from build123d import *

# Parameters (mm, degrees)
F0_W     = 108.1513464451
F0_H     = 106.336735189
F1_DEPTH = 25.4
F2_R     = 30.7442953742
F3_DEPTH = 25.401
F4_R     = 45.0892018552
F4_R_2   = 30.7442953742
F5_DEPTH = 25.4


with BuildPart() as f1:
    # F0 (on Front) → F1 (new body)
    with BuildSketch(Plane.XZ):
        Rectangle(F0_W, F0_H)
    extrude(amount=F1_DEPTH)

    # F2 (on face) → F3 (cut, through all)
    with BuildSketch(Plane.XZ.offset(25.4)):
        Circle(F2_R)
    extrude(amount=-F3_DEPTH, mode=Mode.SUBTRACT)

    # F4 (on face) → F5 (join)
    with BuildSketch(Plane.XZ.offset(25.4)):
        Circle(F4_R)
        Circle(F4_R_2, mode=Mode.SUBTRACT)
    extrude(amount=F5_DEPTH)


solid = f1.part
Part model, mm, in its own coordinate system. A direction names the side the tool comes from. Round coordinates to 2 decimals unless told otherwise and drop trailing zeros. Write each loop counter-clockwise with the first axis right and the second up, starting at its lowest first coordinate (ties: lowest second). Pieces come first, ordered by that corner, then holes. Notation, with made-up numbers: M 14,13 L 26,13 A26 cw 26,41 Z; hole C 63,64.25 d7. An arc over 180 degrees is marked long. Return JSON: item names as keys, results as strings. Group by question number.
(1) Drill centre lines: probe 1 along Z at (x, y) = (0, -40.25); probe 2 along X at (y, z) = (-37, 1); probe 3 along Z at (x, y) = (0, -11). Where is each one in solid material? Low to high.
(2) Which spindle directions (+Z, -Z, +X, -X, +Y, -Y) get a long thin tool onto all of the face, cutting with end or side? Do faces 1 (the face through (-1, -25.4, -47)), 2 (the face through (54.076, -13, -1)). Say none if no direction does.
(3) Saw through at B-B on z = 0. Write the cut outline in (x, y).
(4) Saw through at C-C on y = -16. Write the cut outline in (x, z), then the cut area to 3 significant figures.
(5) Pin check, flat tips, straight feed: pin 1 Ø8 at (y, z) = (-41.5, -11) entering from +X; pin 2 Ø1.5 at (x, y) = (14, -40.5) entering from -Z; pin 3 Ø2 at (y, z) = (-41, 27.5) entering from -X. Stop position of each tip, or through.
(6) Saw through at D-D on z = 39. Write the cut outline in (x, y).
(7) Saw through at A-A on x = 0. Write the cut outline in (y, z).
Returned:
{
 "1": {"probe 1": "-45.09 to -30.74, 30.74 to 45.09", "probe 2": "-45.08 to -30.73, 30.73 to 45.08", "probe 3": "-53.17 to -30.74, 30.74 to 53.17"},
 "2": {"face 1": "-Y", "face 2": "+Z, -Z, +X, +Y, -Y"},
 "3": {"outline": "M -54.08,-25.4 L -45.09,-25.4 L -45.09,-50.8 L -30.74,-50.8 L -30.74,0 L -54.08,0 Z; M 30.74,-50.8 L 45.09,-50.8 L 45.09,-25.4 L 54.08,-25.4 L 54.08,0 L 30.74,0 Z"},
 "4": {"outline": "M -54.08,-53.17 L 54.08,-53.17 L 54.08,53.17 L -54.08,53.17 Z; hole C 0,0 d61.49", "area": "8,530 mm²"},
 "5": {"pin 1": "x = 44.54", "pin 2": "z = -43.1", "pin 3": "x = -36.48"},
 "6": {"outline": "M -54.08,-25.4 L -22.63,-25.4 L -22.63,-50.8 L 22.63,-50.8 L 22.63,-25.4 L 54.08,-25.4 L 54.08,0 L -54.08,0 Z"},
 "7": {"outline": "M -50.8,-45.09 L -25.4,-45.09 L -25.4,-53.17 L 0,-53.17 L 0,-30.74 L -50.8,-30.74 Z; M -50.8,30.74 L 0,30.74 L 0,53.17 L -25.4,53.17 L -25.4,45.09 L -50.8,45.09 Z"}
}
